Check sheet for the modelled part. Datum: model origin and axes. Units: mm. Coordinates: 2 decimals unless noted, no trailing zeros. Loops run counter-clockwise (first coordinate to the right, second up) from the corner with the lowest first, then second, coordinate; pieces in that order, holes last. Notation, with made-up numbers: (66, 77) -> (116, 77) arc R8 cw to (116, 82) -> close; hole circle Ø6 at (-34, 20). An arc over 180 degrees is marked (long way). Use one line per item in the form item = value.
Autodesk Inventor part; units mm, degrees
ref_plane "YZ Plane" through (0, 0, 0) normal (1, 0, 0) x (0, 1, 0)
ref_plane "XZ Plane" through (0, 0, 0) normal (0, 1, 0) x (-1, 0, 0)
ref_plane "XY Plane" through (0, 0, 0) normal (0, 0, 1) x (1, 0, 0)
sketch "Sketch1" plane through (0, 0, 0) normal (1, 0, 0) x (0, 1, 0)
  circle A0 centre (0, 0) radius 13
  dimension "d0" = 26
extrude "Extrusion1" add sketch "Sketch1" along normal blind 14.5
sketch "Sketch2" plane through (0, 0, 0) normal (-1, 0, 0) x (0, 0, 1)
  circle A0 centre (0, 0) radius 13
  circle A1 centre (0, 0) radius 11.5
  dimension "d3" = 23
extrude "Extrusion2" cut sketch "Sketch2" against normal blind 12.5 contours A1
sketch "Sketch3" plane through (14.5, 0, 0) normal (1, 0, 0) x (0, 0, -1)
  circle A0 centre (0, 0) radius 13
  circle A1 centre (0, 0) radius 10.1
  dimension "d6" = 20.2
extrude "Extrusion3" cut sketch "Sketch3" against normal through all contours A1
sketch "Sketch4" plane through (14.5, 0, 0) normal (1, 0, 0) x (0, 0, -1)
  circle A0 centre (0, 0) radius 10.1
  circle A1 centre (0, 0) radius 13
  circle A2 centre (0, 0) radius 10.1
  line L0 (-1.1, -10.0399) -> (-1.1, -12.2399)
  line L1 (-1.1, -12.2399) -> (1.1, -12.2399)
  line L2 (1.1, -12.2399) -> (1.1, -10.0399)
  dimension "d9" = 2.2
extrude "Extrusion4" cut sketch "Sketch4" against normal through all contours A0 L2 L1 L0
properties part number "Button-NUC-Mount"
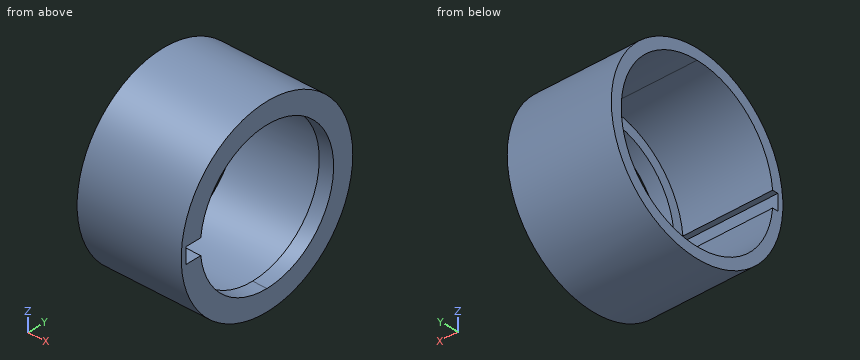
(1) Scan lines: line 1 along Z through (x, y) = (7.25, 0); line 2 along Z through (x, y) = (10, -11.5); line 3 along Y through (x, z) = (11.25, -5.25). Record each from-to range of solid material in increasing order.
Established:
line_1 = -13 to -11.5, 11.5 to 13
line_2 = -6.06 to -1.1, 1.1 to 6.06
line_3 = -11.89 to -10.23, 10.23 to 11.89
(2) Section check C-C, the plane x = 7. Record the boundary of the cut face in (y, z), plus the area to 3 significant figures.
Established:
outline = circle Ø26 at (0, 0); hole (-12.24, -1.1) -> (-11.45, -1.1) arc R11.5 ccw (long way) to (-11.45, 1.1) -> (-12.24, 1.1) -> close
area = 114 mm²
(3) Section check B-B, the plane y = 6. Record the boundary of the cut face in (x, z).
Established:
outline = (0, -11.53) -> (14.5, -11.53) -> (14.5, -8.12) -> (12.5, -8.12) -> (12.5, -9.81) -> (0, -9.81) -> close; (0, 9.81) -> (12.5, 9.81) -> (12.5, 8.12) -> (14.5, 8.12) -> (14.5, 11.53) -> (0, 11.53) -> close
(4) Section check D-D, the plane z = -3.25. Record the boundary of the cut face in (x, y).
Established:
outline = (0, -12.59) -> (14.5, -12.59) -> (14.5, -9.56) -> (12.5, -9.56) -> (12.5, -11.03) -> (0, -11.03) -> close; (0, 11.03) -> (12.5, 11.03) -> (12.5, 9.56) -> (14.5, 9.56) -> (14.5, 12.59) -> (0, 12.59) -> close
(5) Go/stop test with flat-tipped pins: P1, Ø1, axis at x = 8, y = -9.5, coming from the +Z side; P2, Ø2.5, axis at x = 10, y = -11, coming from the -Z side; P3, Ø1.8, axis at x = 6.5, y = -11.5, coming from the +Z side; P4, Ø8, axis at x = 9, z = 0.5, coming from the +Y side. Record where each tip stops, or that it passes through.
Established:
P1 = 9.38
P2 = -8.6
P3 = 7.53
P4 = 13
(6) Section check A-A, the plane z = 0. Record the boundary of the cut face in (x, y), plus the area to 3 significant figures.
Established:
outline = (0, -13) -> (14.5, -13) -> (14.5, -12.24) -> (0, -12.24) -> close; (0, 11.5) -> (12.5, 11.5) -> (12.5, 10.1) -> (14.5, 10.1) -> (14.5, 13) -> (0, 13) -> close
area = 35.6 mm²
